```python
from build123d import *

# Parameters (mm, degrees)
ESBO_O1_R                = 82.5
ESBO_O1_R_2              = 14
RESSALTO_EXTRUS_O1_DEPTH = 3
ESBO_O2_R                = 5.925
RESSALTO_EXTRUS_O2_DEPTH = 8
ESBO_O3_R                = 14
RESSALTO_EXTRUS_O3_DEPTH = 3
ESBO_O4_R                = 10
RESSALTO_EXTRUS_O4_DEPTH = 11
ESBO_O5_R                = 3.05
CORTE_EXTRUS_O1_DEPTH    = 1
ESBO_O6_R                = 76.5
RESSALTO_EXTRUS_O5_DEPTH = 2


with BuildPart() as part:
    # Esboço1 → Ressalto-extrusão1 (new body)
    with BuildSketch(Plane.XY):
        Circle(ESBO_O1_R)
        Circle(ESBO_O1_R_2, mode=Mode.SUBTRACT)
    extrude(amount=RESSALTO_EXTRUS_O1_DEPTH)

    # Esboço2 → Ressalto-extrusão2 (add)
    with BuildSketch(Plane(origin=(0, 0, 0), x_dir=(-1, 0, 0), z_dir=(0, 0, -1))):
        with Locations((-55.155254038, 14.383947721)):
            Circle(ESBO_O2_R)
        with Locations((40.034491152, 40.573877288)):
            Circle(ESBO_O2_R)
        with Locations((15.120762886, -54.957825009)):
            Circle(ESBO_O2_R)
    extrude(amount=RESSALTO_EXTRUS_O2_DEPTH)

    # Esboço3 → Ressalto-extrusão3 (add)
    with BuildSketch(Plane.XY.offset(3)):
        Circle(ESBO_O3_R)
    extrude(amount=-RESSALTO_EXTRUS_O3_DEPTH)

    # Esboço4 → Ressalto-extrusão4 (add)
    with BuildSketch(Plane.XY.offset(3)):
        Circle(ESBO_O4_R)
    extrude(amount=-RESSALTO_EXTRUS_O4_DEPTH)

    # Esboço5 → Corte-extrusão1 (cut)
    with BuildSketch(Plane(origin=(0, 0, -8), x_dir=(-1, 0, 0), z_dir=(0, 0, -1))):
        Circle(ESBO_O5_R)
    extrude(amount=-CORTE_EXTRUS_O1_DEPTH, mode=Mode.SUBTRACT)

    # Esboço6 → Ressalto-extrusão5 (add)
    with BuildSketch(Plane.XY.offset(3)):
        Circle(ESBO_O6_R)
    extrude(amount=RESSALTO_EXTRUS_O5_DEPTH)


solid = part.part
```
The model under review builds one solid part; all positions refer to its coordinate system, in mm. A direction names the side the tool comes from. Give positions to 0.01 mm unless a question says otherwise; leave off trailing zeros. Write each loop counter-clockwise with the first axis right and the second up, starting at its lowest first coordinate (ties: lowest second). Pieces come first, ordered by that corner, then holes. Notation, with made-up numbers: (51.5, 15) -> (69.5, 15) arc R15 cw to (69.5, 44) -> close; hole circle Ø5 at (-5.5, 64.25). An arc over 180 degrees is marked (long way). Answer in a Markdown table with one row per item.
1) Tool access review of faces 1 (the cylindrical face through (-17.88, -80.54, 1.48)), 2 (the flat face through (0, 0, -7)), 3 (the flat face through (73, -24, 3)): name each direction out of +Z, -Z, +X, -X, +Y, -Y from which nothing blocks a thin tool from reaching the whole face with its end or side.
Worked answers:
| item | result |
|---|---|
| face 1 | +Z, -Z |
| face 2 | -Z |
| face 3 | +Z |
2) Add section D-D on x = 68.5. State the section outline as (y, z) points, plus the area to 3 significant figures.
Worked answers:
| item | result |
|---|---|
| outline | (-45.98, 0) -> (45.98, 0) -> (45.98, 3) -> (34.06, 3) -> (34.06, 5) -> (-34.06, 5) -> (-34.06, 3) -> (-45.98, 3) -> close |
| area | 412 mm² |
3) Add section C-C on z = -4.75. Count the separate pieces of the cut face and the enclosed holes in it, plus the area to 3 significant figures.
Worked answers:
| item | result |
|---|---|
| separate pieces | 4 |
| enclosed holes | 0 |
| area | 645 mm² |
4) Mouldability with a two-part tool opening along X and no side actions: class faces 4 (the cylindrical face through (3.047, 0.134, -7.507)), 5 (the cylindrical face through (-60.708, -46.549, 3.986)), 6 (the flat face through (-15, -55, -8)) as +X half, -X half, draft (parallel to the pull), parting line (faces both ways), or undercut.
Worked answers:
| item | result |
|---|---|
| face 4 | undercut |
| face 5 | parting line |
| face 6 | draft |
5) For L1, parallel to Y at x = 0, z = -7.25; L2, parallel to Z at x = -15.5, y = -63; L3, parallel to Y at x = -62, z = 1.25, list the stretches that pass through material, from the lowest coordinate up. Write a range as [from, to].
Worked answers:
| item | result |
|---|---|
| L1 | [-10, -3.05], [3.05, 10] |
| L2 | [0, 5] |
| L3 | [-54.43, 54.43] |
6) Add section A-A on y = 0. State the section outline as (x, z) points, plus the area to 3 significant figures.
Worked answers:
| item | result |
|---|---|
| outline | (-82.5, 0) -> (-10, 0) -> (-10, -8) -> (-3.05, -8) -> (-3.05, -7) -> (3.05, -7) -> (3.05, -8) -> (10, -8) -> (10, 0) -> (82.5, 0) -> (82.5, 3) -> (76.5, 3) -> (76.5, 5) -> (-76.5, 5) -> (-76.5, 3) -> (-82.5, 3) -> close |
| area | 955 mm² |
7) Clearance check with flat-ended pins moving along their axes: P1, Ø4, axis at y = 33.5, z = -1, coming from the -X side; P2, Ø6.5, axis at x = 1.5, y = 1, coming from the -Z side; P3, Ø4, axis at x = 57.5, z = 1.5, coming from the +Y side. State where each tip first meets the part, or that it passes through.
Worked answers:
| item | result |
|---|---|
| P1 | x = -76.14 |
| P2 | z = -8 |
| P3 | y = 61.04 |
